Verification items for the finished model (mm, model axes). Face numbers are marked on the shaded views. A direction names the side the tool comes from. Give positions to 0.01 mm unless a question says otherwise; leave off trailing zeros. Write each loop counter-clockwise with the first axis right and the second up, starting at its lowest first coordinate (ties: lowest second). Pieces come first, ordered by that corner, then holes. Notation, with made-up numbers: (-12, 21.5) - (41, 21.5) arc R12 ccw to (41, 28.5) - close; hole circle Ø8 at (78.5, -33). An arc over 180 degrees is marked (long way). Answer as a JSON object with one key per item and string values. Group by question number.
Item 1: Tool access check on the marked faces 5, 6 and 7. Record the directions out of +Z, -Z, +X, -X, +Y, -Y that give a thin tool (end or side, any length) a straight path to the whole face; none if there is none.
Item 2: Draft check along Z on the marked faces 1, 2, 3 and 4. Enter one of: +Z half, -Z half, draft (parallel to the pull), parting line (faces both ways), or undercut.
Item 3: Scan lines: line 1 along X through (y, z) = (35, 29.5); line 2 along X through (y, z) = (40.5, -2); line 3 along Z through (x, y) = (9, 37.5). Record each from-to range of solid material in increasing order. Write a range as [from, to].
Item 4: Sectioned sample at A-A, the plane y = 33. Record the boundary of the cut face in (x, z), and give its area (3 significant figures).
Item 5: Go/stop test with flat-tipped pins: pin 1 (17 mm diameter, centred on x = 93.69, z = 93.69, fed in from +Y); pin 2 (6 mm diameter, centred on x = -92, y = 18, fed in from -Z); pin 3 (5 mm diameter, centred on x = -63, y = 45.5, fed in from +Z); pin 4 (6 mm diameter, centred on x = -18.5, z = 40.5, fed in from +Y). Record where each tip stops, or that it passes through.
```python
from build123d import *

# Parameters (mm, degrees)
F2_R            = 7.5
F3_DEPTH        = 25.4
F3_COPIES_COUNT = 4
F4_R            = 12.7


# Not quite as in the source:
# - a pattern or mirror of a feature is missing from the dataset's text; its kind, count and spacing are read off the source's solid


with BuildPart() as f1:
    # F0 (on Right) → F1 (revolve)
    with BuildSketch(Plane.YZ):
        Polygon((23.9776, 150), (3.9878, 150), (3.9878, 114.9985), (0, 114.9985), (0, 81.2514126301), (1.524, 81.2514126301), (1.524, 67.9329782724), (6.2865, 67.9329782724), (6.2865, 40.0177), (21.7932, 40.0177), (21.7932, 45.0088), (50.8, 45.0088), (50.8, 51.3588), (12.7, 54.6921180803), (12.7, 113.4999), (44.1452, 113.4999), (44.1452, 118.2624), (39.37, 118.2624), (39.37, 121.5898), (23.9776, 121.5898), align=None)
    revolve(axis=Axis((0, 63.4710703942, 0), (0, 1, 0)))

    # F2 (on face) → F3 (cut)
    with BuildSketch(Plane.XZ.offset(-3.9878)):
        with Locations((-93.6910121111, 93.6910121111)):
            Circle(F2_R)
        with BuildLine():
            Line((-111.0230386257, 169.054677367), (-111.0230386257, 121.5898))
            Line((-111.0230386257, 121.5898), (-87.8403127041, 121.5898))
            ThreePointArc((-87.8403127041, 121.5898), (0, 150), (87.8403127041, 121.5898))
            Line((87.8403127041, 121.5898), (147.7070748806, 121.5898))
            Line((147.7070748806, 121.5898), (147.7070748806, 169.054677367))
            Line((147.7070748806, 169.054677367), (-111.0230386257, 169.054677367))
        make_face()
        with BuildLine():
            ThreePointArc((87.8403127041, 121.5898), (0, 150), (-87.8403127041, 121.5898))
            Line((-87.8403127041, 121.5898), (87.8403127041, 121.5898))
        make_face()
    f3 = extrude(amount=-F3_DEPTH, mode=Mode.SUBTRACT)

    # F3_copies: F3 ×4 about axis
    f3_copies_axis = Axis((0, 0, 0), (0, 1, 0))
    for i in range(1, F3_COPIES_COUNT):
        add(f3.rotate(f3_copies_axis, i * 360 / F3_COPIES_COUNT), mode=Mode.SUBTRACT)

    # F4
    f4_edges = [f1.edges().sort_by_distance(p)[0] for p in [
        (0, 12.7, -113.4999),
        (0, 12.7, -54.692118),
    ]]
    fillet(f4_edges, radius=F4_R)


solid = f1.part
```
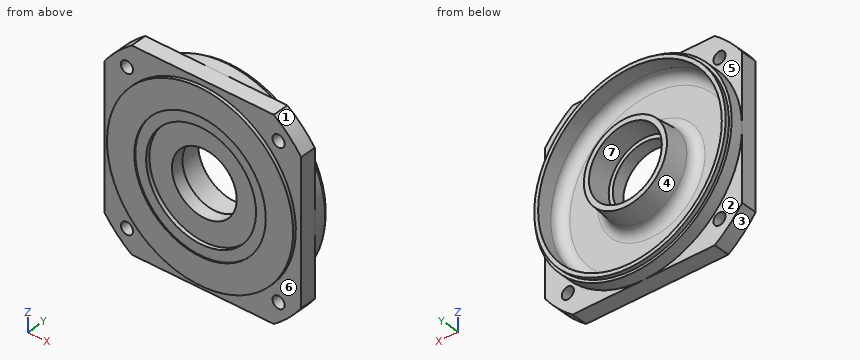
Geometry check:
{
 "1": {"face 5": "+Z, -X, +Y", "face 6": "-Y", "face 7": "+Y"},
 "2": {"face 1": "+Z half", "face 2": "draft", "face 3": "-Z half", "face 4": "undercut"},
 "3": {"line 1": "[-117.96, -109.6], [-43.72, -33.99], [33.99, 43.72], [109.6, 117.96]", "line 2": "[-118.25, -113.48], [-52.22, -44.96], [44.96, 52.22], [113.48, 118.25]", "line 3": "[-121.26, -113.14], [-51.75, -44.1], [44.1, 51.75], [113.14, 121.26]"},
 "4": {"outline": "circle Ø243.18 at (0, 0); circle Ø105.83 at (0, 0); hole circle Ø227 at (0, 0); hole circle Ø90.02 at (0, 0)", "area": "8,410 mm^2"},
 "5": {"pin 1": "y = 23.98", "pin 2": "z = -120.74", "pin 3": "z = 101.38", "pin 4": "y = 50.8"}
}
